Can you work these out from the model? Positions are in its coordinate system, mm. A direction names the side the tool comes from. Give positions to 0.01 mm unless a question says otherwise; leave off trailing zeros. Order: outer loops, then holes, each group sorted by start corner. A loop starts at its lowest first (then second) coordinate and runs counter-clockwise, first axis right, second up. Notation, with made-up numbers: (61.5, 62.5) - (65.5, 62.5) arc R38 cw to (65.5, 100.5) - close; hole circle Ø11 at (-23, -4.5). An arc over 180 degrees is marked (long way). Use one line per item in the form item = value. Start each with the question number.
1) We'd pull the mould along Z, two halves only. Please class faces 1 (the flat face through (20, 15, -2)), 2 (the cylindrical face through (39.43, 12.32, -39.4)), 3 (the cylindrical face through (9.642, 2.465, -22.727)), 4 (the flat face through (18, 25, -1)): released by +Z, released by -Z, zero draft, split by the parting line, or undercut.
2) For pin 1 (8 mm diameter, centred on x = 10.5, z = -9.5, fed in from +Y), with a flat end and sliding along its axis, tell me the tip position at first contact or that it passes through.
3) Suppose I cut it at D-D, the plane x = 5.5. Write out the boundary of the cut face in (y, z), and give its area (3 significant figures).
4) Please list where these lines run through material, in increasing order: probe 1 along X at (y, z) = (1.45, -20); probe 2 along Z at (x, y) = (30, 2.7); probe 3 along X at (y, z) = (16.5, -27.5).
5) Suppose I cut it at A-A, the plane x = 30. Write out the boundary of the cut face in (y, z), and give its area (4 significant figures).
6) Suppose I cut it at C-C, the plane y = 11.25. Write out the boundary of the cut face in (x, z), and give its area (3 significant figures).
7) Which directions (+Z, -Z, +X, -X, +Y, -Y) give clear straight access to the entire face, cutting with the end or side of a thin tool? Please do faces 5 (the flat face through (40, 12, -20)), 6 (the flat face through (20, 15, -38)).
8) Suppose I cut it at B-B, the plane z = -20. Write out the boundary of the cut face in (x, y).
```python
from build123d import *

# Parameters (mm, degrees)
SKETCH1_R           = 2.75
BASE_DEPTH          = 5
SKETCH3_W           = 36
SKETCH3_H           = 36
BOSS_EXTRUDE2_DEPTH = 20


with BuildPart() as part:
    # Sketch1 → base (new body)
    with BuildSketch(Plane(origin=(0, 0, 0), x_dir=(1, 0, 0), z_dir=(0, 1, 0))):
        with BuildLine():
            Line((2, 0), (38, 0))
            ThreePointArc((38, 0), (39.414213562, 0.585786438), (40, 2))
            Line((40, 2), (40, 38))
            ThreePointArc((40, 38), (39.414213562, 39.414213562), (38, 40))
            Line((38, 40), (2, 40))
            ThreePointArc((2, 40), (0.585786438, 39.414213562), (0, 38))
            Line((0, 38), (0, 2))
            ThreePointArc((0, 2), (0.585786438, 0.585786438), (2, 0))
        make_face()
        with Locations((10, 20)):
            Circle(SKETCH1_R, mode=Mode.SUBTRACT)
        with Locations((30, 20)):
            Circle(SKETCH1_R, mode=Mode.SUBTRACT)
    extrude(amount=BASE_DEPTH)

    # Sketch3 → Boss-Extrude2 (add)
    with BuildSketch(Plane(origin=(0, 5, 0), x_dir=(1, 0, 0), z_dir=(0, 1, 0))):
        with BuildLine():
            Line((0, 38), (0, 2))
            ThreePointArc((0, 2), (0.585786438, 0.585786438), (2, 0))
            Line((2, 0), (38, 0))
            ThreePointArc((38, 0), (39.414213562, 0.585786438), (40, 2))
            Line((40, 2), (40, 38))
            ThreePointArc((40, 38), (39.414213562, 39.414213562), (38, 40))
            Line((38, 40), (2, 40))
            ThreePointArc((2, 40), (0.585786438, 39.414213562), (0, 38))
        make_face()
        with Locations((20, 20)):
            Rectangle(SKETCH3_W, SKETCH3_H, mode=Mode.SUBTRACT)
    extrude(amount=BOSS_EXTRUDE2_DEPTH)


solid = part.part
```
Result sheet:
q1.face_1 = undercut
q1.face_2 = released by -Z
q1.face_3 = undercut
q1.face_4 = zero draft
q2.pin_1 = 5
q3.outline = (0, -40) - (25, -40) - (25, -38) - (5, -38) - (5, -2) - (25, -2) - (25, 0) - (0, 0) - close
q3.area = 280 mm²
q4.probe_1 = 0 to 7.25, 12.75 to 27.25, 32.75 to 40
q4.probe_2 = -40 to -22.75, -17.25 to 0
q4.probe_3 = 0 to 2, 38 to 40
q5.outline = (0, -40) - (25, -40) - (25, -38) - (5, -38) - (5, -22.75) - (0, -22.75) - close; (0, -17.25) - (5, -17.25) - (5, -2) - (25, -2) - (25, 0) - (0, 0) - close
q5.area = 252.5 mm²
q6.outline = (0, -38) arc R2 ccw to (2, -40) - (38, -40) arc R2 ccw to (40, -38) - (40, -2) arc R2 ccw to (38, 0) - (2, 0) arc R2 ccw to (0, -2) - close; hole (2, -38) - (38, -38) - (38, -2) - (2, -2) - close
q6.area = 301 mm²
q7.face_5 = +Z, -Z, +X, +Y, -Y
q7.face_6 = +Y
q8.outline = (0, 0) - (7.25, 0) - (7.25, 5) - (2, 5) - (2, 25) - (0, 25) - close; (12.75, 0) - (27.25, 0) - (27.25, 5) - (12.75, 5) - close; (32.75, 0) - (40, 0) - (40, 25) - (38, 25) - (38, 5) - (32.75, 5) - close
